```python
from build123d import *

# Parameters (mm, degrees)
SKETCH_1_R             = 175
EXTRUDE_1_DEPTH        = 3
CUT_EXTRUDE_1_DEPTH    = 3
FILLET_1_R             = 5
FILLET_2_R             = 5
FILLET_3_R             = 5
SKETCH_5_R             = 1.5
CUT_EXTRUDE_4_DEPTH    = 3
SKETCH_6_R             = 1.5
CUT_EXTRUDE_5_DEPTH    = 3
SKETCH_7_W             = 30
SKETCH_7_H             = 108
CUT_EXTRUDE_6_DEPTH    = 3
SKETCH_8_R             = 1.5
CUT_EXTRUDE_7_DEPTH    = 3
SKETCH_9_R             = 1.5
CUT_EXTRUDE_8_DEPTH    = 10
SKETCH_10_R            = 1.6
CUT_EXTRUDE_5158_DEPTH = 10
SKETCH_11_W            = 15
SKETCH_11_H            = 30
CUT_EXTRUDE_10_DEPTH   = 10
SKETCH_19_R            = 1.6
CUT_EXTRUDE_8157_DEPTH = 10
SKETCH_21_R            = 1.5
WEB_DEPTH              = 10
SKETCH_22_R            = 1.5
WEB_2_DEPTH            = 10
SKETCH_28_R            = 1.5
CUT_EXTRUDE_9035_DEPTH = 10
SKETCH_29_R            = 1.5
CUT_EXTRUDE_9316_DEPTH = 10
SKETCH_31_R            = 1.5
CUT_EXTRUDE_9726_DEPTH = 10


with BuildPart() as part:
    # ｽｹｯﾁ1 → ﾎﾞｽ - 押し出し1 (new body)
    with BuildSketch(Plane.XY):
        Circle(SKETCH_1_R)
    extrude(amount=EXTRUDE_1_DEPTH)

    # ｽｹｯﾁ2 → ｶｯﾄ - 押し出し1 (cut)
    with BuildSketch(Plane.XY.offset(3)):
        with BuildLine():
            Line((-60, 115), (0, 115))
            Line((0, 115), (0, 175))
            ThreePointArc((0, 175), (-30.465194158, 172.327803749), (-60, 164.392822228))
            Line((-60, 164.392822228), (-60, 115))
        make_face()
        with BuildLine():
            Line((0, 175), (0, 115))
            Line((0, 115), (60, 115))
            Line((60, 115), (60, 164.392822228))
            ThreePointArc((60, 164.392822228), (30.465194158, 172.327803749), (0, 175))
        make_face()
        with BuildLine():
            Line((0, -175), (0, -115))
            Line((0, -115), (-60, -115))
            Line((-60, -115), (-60, -164.392822228))
            ThreePointArc((-60, -164.392822228), (-30.465194158, -172.327803749), (0, -175))
        make_face()
        with BuildLine():
            Line((60, -115), (0, -115))
            Line((0, -115), (0, -175))
            ThreePointArc((0, -175), (30.465194158, -172.327803749), (60, -164.392822228))
            Line((60, -164.392822228), (60, -115))
        make_face()
    extrude(amount=-CUT_EXTRUDE_1_DEPTH, mode=Mode.SUBTRACT)

    # ﾌｨﾚｯﾄ1
    fillet_1_edges = [part.edges().sort_by_distance(p)[0] for p in [
        (-60, 164.392822228, 1.5),
    ]]
    fillet(fillet_1_edges, radius=FILLET_1_R)

    # ﾌｨﾚｯﾄ2
    fillet_2_edges = [part.edges().sort_by_distance(p)[0] for p in [
        (-60, 115, 1.5),
        (60, 164.392822228, 1.5),
        (60, 115, 1.5),
    ]]
    fillet(fillet_2_edges, radius=FILLET_2_R)

    # ﾌｨﾚｯﾄ3
    fillet_3_edges = [part.edges().sort_by_distance(p)[0] for p in [
        (-60, -115, 1.5),
        (60, -115, 1.5),
        (60, -164.392822228, 1.5),
        (-60, -164.392822228, 1.5),
    ]]
    fillet(fillet_3_edges, radius=FILLET_3_R)

    # ｽｹｯﾁ5 → ｶｯﾄ - 押し出し4 (cut)
    with BuildSketch(Plane.XY.offset(3)):
        with Locations((-100, -115)):
            Circle(SKETCH_5_R)
        with Locations((100, -115)):
            Circle(SKETCH_5_R)
        with Locations((100, 115)):
            Circle(SKETCH_5_R)
        with Locations((-100, 115)):
            Circle(SKETCH_5_R)
    extrude(amount=-CUT_EXTRUDE_4_DEPTH, mode=Mode.SUBTRACT)

    # ｽｹｯﾁ6 → ｶｯﾄ - 押し出し5 (cut)
    with BuildSketch(Plane.XY.offset(3)):
        with Locations((-60, 54)):
            Circle(SKETCH_6_R)
        with Locations((60, 54)):
            Circle(SKETCH_6_R)
        with Locations((-60, -54)):
            Circle(SKETCH_6_R)
        with Locations((60, -54)):
            Circle(SKETCH_6_R)
    extrude(amount=-CUT_EXTRUDE_5_DEPTH, mode=Mode.SUBTRACT)

    # ｽｹｯﾁ7 → ｶｯﾄ - 押し出し6 (cut)
    with BuildSketch(Plane.XY.offset(3)):
        with Locations((-85, 0)):
            Rectangle(SKETCH_7_W, SKETCH_7_H)
    extrude(amount=-CUT_EXTRUDE_6_DEPTH, mode=Mode.SUBTRACT)

    # ｽｹｯﾁ8 → ｶｯﾄ - 押し出し7 (cut)
    with BuildSketch(Plane.XY.offset(3)):
        with Locations((-115, -67)):
            Circle(SKETCH_8_R)
        with Locations((-116.822468618, 0)):
            Circle(SKETCH_8_R)
        with Locations((-115, 67)):
            Circle(SKETCH_8_R)
    extrude(amount=-CUT_EXTRUDE_7_DEPTH, mode=Mode.SUBTRACT)

    # ｽｹｯﾁ9 → ｶｯﾄ - 押し出し8 (cut)
    with BuildSketch(Plane.XY.offset(3)):
        with Locations((-65, 37)):
            Circle(SKETCH_9_R)
        with Locations((20, 41)):
            Circle(SKETCH_9_R)
        with Locations((-65, -38)):
            Circle(SKETCH_9_R)
        with Locations((20, -40)):
            Circle(SKETCH_9_R)
    extrude(amount=-CUT_EXTRUDE_8_DEPTH, mode=Mode.SUBTRACT)

    # ｽｹｯﾁ10 → Cut-Extrude 5158 (cut)
    with BuildSketch(Plane.XY.offset(3)):
        with Locations((111.643659725, -125.921059639)):
            Circle(SKETCH_10_R)
        with Locations((122.679794489, -115.037952538)):
            Circle(SKETCH_10_R)
        with Locations((168, 7.75)):
            Circle(SKETCH_10_R)
        with Locations((168, -7.75)):
            Circle(SKETCH_10_R)
        with Locations((111.56768007, 125.844011632)):
            Circle(SKETCH_10_R)
        with Locations((122.679794489, 115.037952538)):
            Circle(SKETCH_10_R)
    extrude(amount=-CUT_EXTRUDE_5158_DEPTH, mode=Mode.SUBTRACT)

    # ｽｹｯﾁ11 → ｶｯﾄ - 押し出し10 (cut)
    with BuildSketch(Plane.XY.offset(3)):
        with Locations((81.317279836, 81.317279836)):
            Rectangle(SKETCH_11_W, SKETCH_11_H)
        with Locations((81.317279836, -81.317279836)):
            Rectangle(SKETCH_11_W, SKETCH_11_H)
    extrude(amount=-CUT_EXTRUDE_10_DEPTH, mode=Mode.SUBTRACT)

    # ｽｹｯﾁ19 → Cut-Extrude 8157 (cut)
    with BuildSketch(Plane.XY.offset(3)):
        with Locations((-111.442990249, 125.715790275)):
            Circle(SKETCH_19_R)
        with Locations((-122.555104667, 114.909731181)):
            Circle(SKETCH_19_R)
        with Locations((-167.821147356, 7.75)):
            Circle(SKETCH_19_R)
        with Locations((-167.821147356, -7.75)):
            Circle(SKETCH_19_R)
        with Locations((-122.555104667, -114.909731181)):
            Circle(SKETCH_19_R)
        with Locations((-111.442990249, -125.715790275)):
            Circle(SKETCH_19_R)
    extrude(amount=-CUT_EXTRUDE_8157_DEPTH, mode=Mode.SUBTRACT)

    # ｽｹｯﾁ21 → Web (cut)
    with BuildSketch(Plane.XY.offset(3)):
        with Locations((-145, 25)):
            Circle(SKETCH_21_R)
        with Locations((-145, -25)):
            Circle(SKETCH_21_R)
    extrude(amount=-WEB_DEPTH, mode=Mode.SUBTRACT)

    # ｽｹｯﾁ22 → Web 2 (cut)
    with BuildSketch(Plane.XY.offset(3)):
        with Locations((125, 25)):
            Circle(SKETCH_22_R)
        with Locations((125, -25)):
            Circle(SKETCH_22_R)
    extrude(amount=-WEB_2_DEPTH, mode=Mode.SUBTRACT)

    # ｽｹｯﾁ28 → Cut-Extrude 9035 (cut)
    with BuildSketch(Plane.XY.offset(3)):
        with Locations((40, 45)):
            Circle(SKETCH_28_R)
        with Locations((90, 45)):
            Circle(SKETCH_28_R)
        with Locations((40, -45)):
            Circle(SKETCH_28_R)
        with Locations((90, -45)):
            Circle(SKETCH_28_R)
    extrude(amount=-CUT_EXTRUDE_9035_DEPTH, mode=Mode.SUBTRACT)

    # ｽｹｯﾁ29 → Cut-Extrude 9316 (cut)
    with BuildSketch(Plane.XY.offset(3)):
        with Locations((80, 125)):
            Circle(SKETCH_29_R)
        with Locations((80, 110)):
            Circle(SKETCH_29_R)
        with Locations((80, -110)):
            Circle(SKETCH_29_R)
        with Locations((80, -125)):
            Circle(SKETCH_29_R)
    extrude(amount=-CUT_EXTRUDE_9316_DEPTH, mode=Mode.SUBTRACT)

    # ｽｹｯﾁ31 → Cut-Extrude 9726 (cut)
    with BuildSketch(Plane.XY.offset(3)):
        with Locations((-92, 130)):
            Circle(SKETCH_31_R)
        with Locations((-75, 130)):
            Circle(SKETCH_31_R)
        with Locations((75, 130)):
            Circle(SKETCH_31_R)
        with Locations((92, 130)):
            Circle(SKETCH_31_R)
        with Locations((92, -130)):
            Circle(SKETCH_31_R)
        with Locations((75, -130)):
            Circle(SKETCH_31_R)
        with Locations((-75, -130)):
            Circle(SKETCH_31_R)
        with Locations((-92, -130)):
            Circle(SKETCH_31_R)
    extrude(amount=-CUT_EXTRUDE_9726_DEPTH, mode=Mode.SUBTRACT)


solid = part.part
```
Model file for the job. Use its own axes, mm. Round coordinates to 2 decimals unless told otherwise and drop trailing zeros. Write each loop counter-clockwise with the first axis right and the second up, starting at its lowest first coordinate (ties: lowest second). Pieces come first, ordered by that corner, then holes. Notation, with made-up numbers: (45.5, 3) - (66.5, 3) arc R33 cw to (66.5, 42) - close; hole circle Ø1 at (-15.5, 8). An arc over 180 degrees is marked (long way). Use CSV: the item, a comma, the result in double quotes. Start each with the question number.
Item 1: Drill centre lines: L1, parallel to Y at x = -65, z = 2.35; L2, parallel to Y at x = -75, z = 1.05; L3, parallel to Y at x = 75, z = 1.85. Where is each one in solid material? Low to high. Write a range as [from, to].
Item 2: Band-saw the part on A-A (y = 139). Write the cut outline in (x, z), and give its area (3 significant figures).
Item 3: Band-saw the part on C-C (z = 0.5). State how many separate pieces and enclosed holes the cut face has, and give its area (3 significant figures).
Item 4: Pin check, flat tips, straight feed: P1, Ø1.9, axis at x = -111.44, y = -125.72, coming from the -Z side; P2, Ø1.5, axis at y = -107, z = 1.5, coming from the -X side; P3, Ø1, axis at x = 69, z = 2.5, coming from the +Y side; P4, Ø1.5, axis at y = 62.5, z = 0.5, coming from the -X side. Stop position of each tip, or through.
Item 5: Band-saw the part on B-B (x = -82). Write the cut outline in (y, z), and give its area (3 significant figures).
Item 6: Band-saw the part on D-D (x = -135). Write the cut outline in (y, z), and give its area (3 significant figures).
Checked values:
1,L1,"y = [-162.08, -39.5], [-36.5, 35.5], [38.5, 162.08]"
1,L2,"y = [-158.11, -131.5], [-128.5, -54], [54, 128.5], [131.5, 158.11]"
1,L3,"y = [-158.11, -131.5], [-128.5, -96.32], [-66.32, 66.32], [96.32, 128.5], [131.5, 158.11]"
2,outline,"(-106.32, 0) - (-60, 0) - (-60, 3) - (-106.32, 3) - close; (60, 0) - (106.32, 0) - (106.32, 3) - (60, 3) - close"
2,area,"278 mm²"
3,separate pieces,"1"
3,enclosed holes,"50"
3,area,"78,100 mm²"
4,P1,"passes through"
4,P2,"stops at x = -139.05"
4,P3,"stops at y = 161.04"
4,P4,"stops at x = -163.74"
5,outline,"(-154.6, 0) - (-54, 0) - (-54, 3) - (-154.6, 3) - close; (54, 0) - (154.6, 0) - (154.6, 3) - (54, 3) - close"
5,area,"604 mm²"
6,outline,"(-111.36, 0) - (111.36, 0) - (111.36, 3) - (-111.36, 3) - close"
6,area,"668 mm²"
